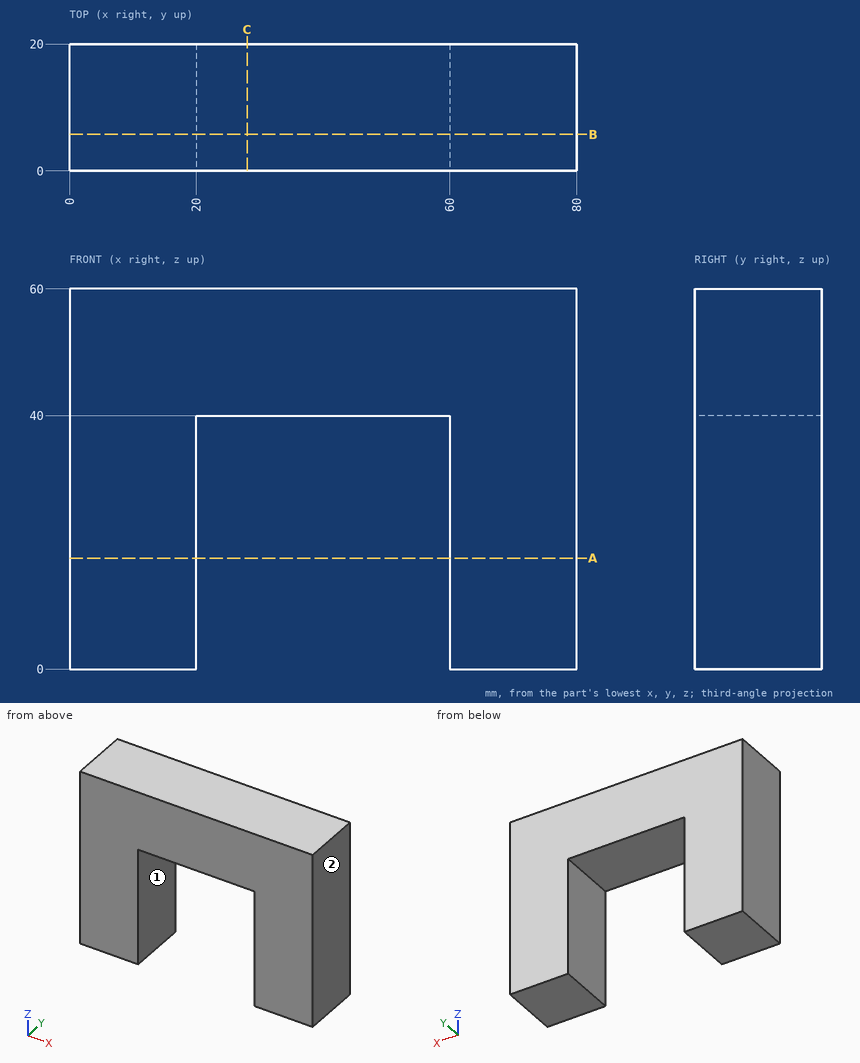
Drawing for the job (mm, zero at the part's lowest x, y, z). A direction names the side the tool comes from. Round coordinates to 2 decimals unless told otherwise and drop trailing zeros. Write each loop counter-clockwise with the first axis right and the second up, starting at its lowest first coordinate (ties: lowest second). Pieces come first, ordered by that corner, then holes. Notation, with made-up numbers: M -4,-36.5 L 45,-36.5 A22 cw 45,-16.5 Z; hole C -21.75,-4 d2. An arc over 180 degrees is marked long. One line per question, with ' | ' between items.
1. Cut at C-C on x = 28. Write the cut outline in (y, z).
Working result:
outline: M 0,40 L 20,40 L 20,60 L 0,60 Z
2. Which spindle directions (+Z, -Z, +X, -X, +Y, -Y) get a long thin tool onto all of the face, cutting with end or side? Do the marked faces 1 and 2. Say none if no direction does.
Working result:
face 1: -Z, +Y, -Y | face 2: +Z, -Z, +X, +Y, -Y
3. Cut at B-B on y = 5.75. Write the cut outline in (x, z), and give its area (3 significant figures).
Working result:
outline: M 0,0 L 20,0 L 20,40 L 60,40 L 60,0 L 80,0 L 80,60 L 0,60 Z | area: 3,200 mm2
4. Pin check, flat tip, straight feed: pin 1 Ø5 at (x, y) = (25.5, 12) entering from -Z. Stop position of the tip, or through.
Working result:
pin 1: z = 40
5. Probe L1, parallel to X at y = 3.5, z = 22.5; L2, parallel to Z at x = 39.5, y = 18.75. List the from-to ranges inside material, lowest first. Write a range as from..to.
Working result:
L1: 0..20, 60..80 | L2: 40..60
6. Cut at A-A on z = 17.5. Write the cut outline in (x, y), and give its area (3 significant figures).
Working result:
outline: M 0,0 L 20,0 L 20,20 L 0,20 Z; M 60,0 L 80,0 L 80,20 L 60,20 Z | area: 800 mm2
